Read the model definition and answer for the solid it produces. Units are mm, in the model's axes. Coordinates: 2 decimals unless noted, no trailing zeros. Write each loop counter-clockwise with the first axis right and the second up, starting at its lowest first coordinate (ties: lowest second). Pieces come first, ordered by that corner, then holes. Notation, with made-up numbers: (-21.5, 8.25) - (11.5, 8.25) arc R14 cw to (11.5, 26.25) - close; hole circle Ø4 at (64.5, 64). An arc over 180 degrees is marked (long way). Use a Markdown table: item, result.
from build123d import *

# Parameters (mm, degrees)
SKETCH_1_R      = 0.3
EXTRUDE_4_DEPTH = 1


with BuildPart() as part:
    # 草图1 → 凸台-拉伸4 (new body)
    with BuildSketch(Plane.XY):
        with BuildLine():
            Line((-0.100008903, 1.994986542), (-14.006783195, 0.597177449))
            ThreePointArc((-14.006783195, 0.597177449), (-14.603960644, 0), (-14.006783195, -0.597177449))
            Line((-14.006783195, -0.597177449), (-0.100008903, -1.994986542))
            ThreePointArc((-0.100008903, -1.994986542), (0, -2), (0.100008903, -1.994986542))
            Line((0.100008903, -1.994986542), (14.006783195, -0.597177449))
            ThreePointArc((14.006783195, -0.597177449), (14.595169998, 0), (14.006783195, 0.597177449))
            Line((14.006783195, 0.597177449), (0.100008903, 1.994986542))
            ThreePointArc((0.100008903, 1.994986542), (0, 2), (-0.100008903, 1.994986542))
        make_face()
        with Locations((0, -1)):
            Circle(SKETCH_1_R, mode=Mode.SUBTRACT)
        with Locations((-14.006783195, 0)):
            Circle(SKETCH_1_R, mode=Mode.SUBTRACT)
        with BuildLine():
            ThreePointArc((0, -0.3), (-0.3, 0), (0, 0.3))
            ThreePointArc((0, 0.3), (0.3, 0), (0, -0.3))
        make_face(mode=Mode.SUBTRACT)
        with Locations((0, 1)):
            Circle(SKETCH_1_R, mode=Mode.SUBTRACT)
        with Locations((14.006783195, 0)):
            Circle(SKETCH_1_R, mode=Mode.SUBTRACT)
    extrude(amount=EXTRUDE_4_DEPTH)


solid = part.part
(1) A cutting plane is placed at D-D, the plane y = 1.65. Write down the section's boundary in (x, z), and give its area (3 significant figures).
Report:
| item | result |
|---|---|
| outline | (-3.53, 0) - (3.53, 0) - (3.53, 1) - (-3.53, 1) - close |
| area | 7.06 mm² |
(2) Straight lines are drawn through the part: L1, parallel to X at y = -0.25, z = 0.9; L2, parallel to X at y = -0.4, z = 0.8; L3, parallel to Y at x = 7.5, z = 0.6. For each, find the intervals that lie inside material, in ascending order.
Report:
| item | result |
|---|---|
| L1 | x = -14.55 to -14.17, -13.84 to -0.17, 0.17 to 13.84, 14.17 to 14.54 |
| L2 | x = -14.45 to 14.44 |
| L3 | y = -1.25 to 1.25 |
(3) A cutting plane is placed at B-B, the plane z = 0.5. Write down the section's boundary in (x, y), and give its area (3 significant figures).
Report:
| item | result |
|---|---|
| outline | (-14.01, -0.6) - (-0.1, -1.99) arc R1 ccw to (0.1, -1.99) - (14.01, -0.6) arc R0.6 ccw to (14.01, 0.6) - (0.1, 1.99) arc R1 ccw to (-0.1, 1.99) - (-14.01, 0.6) arc R0.6 ccw to start; hole circle Ø0.6 at (-14.01, 0); hole circle Ø0.6 at (0, -1); hole circle Ø0.6 at (0, 0); hole circle Ø0.6 at (0, 1); hole circle Ø0.6 at (14.01, 0) |
| area | 72.6 mm² |
(4) A cutting plane is placed at C-C, the plane x = -3.25. Write down the section's boundary in (y, z), and give its area (3 significant figures).
Report:
| item | result |
|---|---|
| outline | (-1.68, 0) - (1.68, 0) - (1.68, 1) - (-1.68, 1) - close |
| area | 3.36 mm² |
(5) A cutting plane is placed at A-A, the plane y = 0. Write down the section's boundary in (x, z).
Report:
| item | result |
|---|---|
| outline | (-14.6, 0) - (-14.31, 0) - (-14.31, 1) - (-14.6, 1) - close; (-13.71, 0) - (-0.3, 0) - (-0.3, 1) - (-13.71, 1) - close; (0.3, 0) - (13.71, 0) - (13.71, 1) - (0.3, 1) - close; (14.31, 0) - (14.6, 0) - (14.6, 1) - (14.31, 1) - close |
